```python
from build123d import *

# Parameters (mm, degrees)
SKETCH1_W               = 60
SKETCH1_H               = 40
BOSS_EXTRUDE1_DEPTH     = 27
SKETCH2_W               = 8
SKETCH2_H               = 3
CUT_EXTRUDE1_DEPTH      = 1
CUT_EXTRUDE1_DRAFT      = -35
MIRROR1_COPY_1_SKETCH_W = 8
MIRROR1_COPY_1_SKETCH_H = 3
MIRROR1_COPY_1_DEPTH    = 1
MIRROR1_COPY_1_DRAFT    = -35
MIRROR2_COPY_1_SKETCH_W = 8
MIRROR2_COPY_1_SKETCH_H = 3
MIRROR2_COPY_1_DEPTH    = 1
MIRROR2_COPY_1_DRAFT    = -35
MIRROR2_COPY_2_SKETCH_W = 8
MIRROR2_COPY_2_SKETCH_H = 3
MIRROR2_COPY_2_DEPTH    = 1
MIRROR2_COPY_2_DRAFT    = -35
BOSS_EXTRUDE2_START     = 27
SKETCH1_3_W             = 60
SKETCH1_3_H             = 40
BOSS_EXTRUDE2_DEPTH     = 2
SKETCH3_W               = 21.960696684
SKETCH3_H               = 27.5
CUT_EXTRUDE2_DEPTH      = 2
SKETCH3_3_R             = 2.5
SKETCH3_3_R_2           = 1.4
SKETCH3_3_R_3           = 2.519651658
BOSS_EXTRUDE3_DEPTH     = 5
SKETCH4_W               = 20
SKETCH4_H               = 27
BOSS_EXTRUDE4_DEPTH     = 8
CHAMFER1_SIZE           = 5
CHAMFER1_SIZE_2         = 8.660254038
SKETCH5_W               = 8
SKETCH5_H               = 20
CUT_EXTRUDE3_DEPTH      = 25
SKETCH6_W               = 12
SKETCH6_H               = 40
CUT_EXTRUDE5_DEPTH      = 1.5


with BuildPart() as part:
    # Sketch1 → Boss-Extrude1 (new body)
    with BuildSketch(Plane(origin=(0, 0, 0), x_dir=(1, 0, 0), z_dir=(0, 1, 0))):
        Polygon((-32, 22), (-20, 22), (-20, 21), (-12, 21), (-12, 22), (12, 22), (12, 21), (20, 21), (20, 22), (32, 22), (32, -22), (20, -22), (20, -21), (12, -21), (12, -22), (-12, -22), (-12, -21), (-20, -21), (-20, -22), (-32, -22), align=None)
        Rectangle(SKETCH1_W, SKETCH1_H, mode=Mode.SUBTRACT)
    extrude(amount=BOSS_EXTRUDE1_DEPTH)


with BuildPart() as cut_extrude1_tool:
    # Sketch2 → Cut-Extrude1 (with draft: the straight prism first)
    with BuildSketch(Plane.XY.offset(21)):
        with Locations((-16, 5.5)):
            Rectangle(SKETCH2_W, SKETCH2_H)
    extrude(amount=-CUT_EXTRUDE1_DEPTH)
    # Cut-Extrude1: the draft: its side faces are tilted about the plane it starts from
    cut_extrude1_sides = [cut_extrude1_tool.faces().sort_by_distance(p)[0] for p in [
        (-20, 5.5, 20.5),
        (-16, 4, 20.5),
        (-12, 5.5, 20.5),
        (-16, 7, 20.5),
    ]]
    draft(cut_extrude1_sides, Plane.XY.offset(21), CUT_EXTRUDE1_DRAFT)


with BuildPart() as part_1:
    add(part.part)

    # Cut-Extrude1: cut by cut_extrude1_tool
    add(cut_extrude1_tool.part, mode=Mode.SUBTRACT)


with BuildPart() as mirror1_copy_1_tool:
    # Mirror1 copy 1 sketch → Mirror1 copy 1 (with draft: the straight prism first)
    with BuildSketch(Plane(origin=(0, 0, 21), x_dir=(-1, 0, 0), z_dir=(0, 0, 1))):
        with Locations((-16, -5.5)):
            Rectangle(MIRROR1_COPY_1_SKETCH_W, MIRROR1_COPY_1_SKETCH_H)
    extrude(amount=-MIRROR1_COPY_1_DEPTH)
    # Mirror1 copy 1: the draft: its side faces are tilted about the plane it starts from
    mirror1_copy_1_sides = [mirror1_copy_1_tool.faces().sort_by_distance(p)[0] for p in [
        (20, 5.5, 20.5),
        (16, 4, 20.5),
        (12, 5.5, 20.5),
        (16, 7, 20.5),
    ]]
    draft(mirror1_copy_1_sides, Plane(origin=(0, 0, 21), x_dir=(-1, 0, 0), z_dir=(0, 0, 1)), MIRROR1_COPY_1_DRAFT)


with BuildPart() as part_2:
    add(part_1.part)

    # Mirror1 copy 1: cut by mirror1_copy_1_tool
    add(mirror1_copy_1_tool.part, mode=Mode.SUBTRACT)


with BuildPart() as mirror2_copy_1_tool:
    # Mirror2 copy 1 sketch → Mirror2 copy 1 (with draft: the straight prism first)
    with BuildSketch(Plane(origin=(0, 0, -21), x_dir=(1, 0, 0), z_dir=(0, 0, -1))):
        with Locations((-16, -5.5)):
            Rectangle(MIRROR2_COPY_1_SKETCH_W, MIRROR2_COPY_1_SKETCH_H)
    extrude(amount=-MIRROR2_COPY_1_DEPTH)
    # Mirror2 copy 1: the draft: its side faces are tilted about the plane it starts from
    mirror2_copy_1_sides = [mirror2_copy_1_tool.faces().sort_by_distance(p)[0] for p in [
        (-20, 5.5, -20.5),
        (-16, 4, -20.5),
        (-12, 5.5, -20.5),
        (-16, 7, -20.5),
    ]]
    draft(mirror2_copy_1_sides, Plane(origin=(0, 0, -21), x_dir=(1, 0, 0), z_dir=(0, 0, -1)), MIRROR2_COPY_1_DRAFT)


with BuildPart() as part_3:
    add(part_2.part)

    # Mirror2 copy 1: cut by mirror2_copy_1_tool
    add(mirror2_copy_1_tool.part, mode=Mode.SUBTRACT)


with BuildPart() as mirror2_copy_2_tool:
    # Mirror2 copy 2 sketch → Mirror2 copy 2 (with draft: the straight prism first)
    with BuildSketch(Plane(origin=(0, 0, -21), x_dir=(-1, 0, 0), z_dir=(0, 0, -1))):
        with Locations((-16, 5.5)):
            Rectangle(MIRROR2_COPY_2_SKETCH_W, MIRROR2_COPY_2_SKETCH_H)
    extrude(amount=-MIRROR2_COPY_2_DEPTH)
    # Mirror2 copy 2: the draft: its side faces are tilted about the plane it starts from
    mirror2_copy_2_sides = [mirror2_copy_2_tool.faces().sort_by_distance(p)[0] for p in [
        (20, 5.5, -20.5),
        (16, 4, -20.5),
        (12, 5.5, -20.5),
        (16, 7, -20.5),
    ]]
    draft(mirror2_copy_2_sides, Plane(origin=(0, 0, -21), x_dir=(-1, 0, 0), z_dir=(0, 0, -1)), MIRROR2_COPY_2_DRAFT)


with BuildPart() as part_4:
    add(part_3.part)

    # Mirror2 copy 2: cut by mirror2_copy_2_tool
    add(mirror2_copy_2_tool.part, mode=Mode.SUBTRACT)

    # Sketch1<3> → Boss-Extrude2 (add)
    with BuildSketch(Plane(origin=(0, 0, 0), x_dir=(1, 0, 0), z_dir=(0, 1, 0)).offset(BOSS_EXTRUDE2_START)):
        Rectangle(SKETCH1_3_W, SKETCH1_3_H)
    extrude(amount=-BOSS_EXTRUDE2_DEPTH)

    # Sketch3 → Cut-Extrude2 (cut)
    with BuildSketch(Plane.XZ.offset(-25)):
        with Locations((0.5, 4.25)):
            Rectangle(SKETCH3_W, SKETCH3_H)
    extrude(amount=-CUT_EXTRUDE2_DEPTH, mode=Mode.SUBTRACT)

    # Sketch3<3> → Boss-Extrude3 (add)
    # profile 1 of 4: a face of its own
    with BuildSketch(Plane.XZ.offset(-25)):
        with Locations(Location((-13, 15.25, 0), (0, 0, 90))):
            Circle(SKETCH3_3_R)
        with Locations(Location((-13, 15.25, 0), (0, 0, 270))):
            Circle(SKETCH3_3_R_2, mode=Mode.SUBTRACT)
    # profile 2 of 4: a face of its own
    with BuildSketch(Plane.XZ.offset(-25)):
        with Locations((-13, -6.75)):
            Circle(SKETCH3_3_R_3)
        with Locations(Location((-13, -6.75, 0), (0, 0, 270))):
            Circle(SKETCH3_3_R_2, mode=Mode.SUBTRACT)
    # profile 3 of 4: a face of its own
    with BuildSketch(Plane.XZ.offset(-25)):
        with Locations(Location((14, -6.75, 0), (0, 0, 180))):
            Circle(SKETCH3_3_R_3)
        with Locations(Location((14, -6.75, 0), (0, 0, 270))):
            Circle(SKETCH3_3_R_2, mode=Mode.SUBTRACT)
    # profile 4 of 4: a face of its own
    with BuildSketch(Plane.XZ.offset(-25)):
        with Locations(Location((14, 15.25, 0), (0, 0, 90))):
            Circle(SKETCH3_3_R)
        with Locations(Location((14, 15.25, 0), (0, 0, 270))):
            Circle(SKETCH3_3_R_2, mode=Mode.SUBTRACT)
    extrude(amount=BOSS_EXTRUDE3_DEPTH)

    # Sketch4 → Boss-Extrude4 (add)
    with BuildSketch(Plane(origin=(32, 0, 0), x_dir=(0, 0, -1), z_dir=(1, 0, 0))):
        with Locations((10, 13.5)):
            Rectangle(SKETCH4_W, SKETCH4_H)
    extrude(amount=BOSS_EXTRUDE4_DEPTH)

    # Chamfer1
    # the kernel refuses this chamfer: 8.660254038, 5 mm, written as the material it adds along each edge
    with BuildSketch(Plane(origin=(32, 27, -20), x_dir=(-0.05789386240267251, 0, -0.9983227437537924), z_dir=(0, -1, 0))) as chamfer1_piece_1_section:
        Polygon((CHAMFER1_SIZE * 0.998322743754, CHAMFER1_SIZE * 0.0578938624027), (-CHAMFER1_SIZE_2 * 0.0578938624016, CHAMFER1_SIZE_2 * 0.998322743736), (0, 0), align=None)
    chamfer1_piece_1 = extrude(amount=27, mode=Mode.PRIVATE)
    chamfer1_piece_1 = split(chamfer1_piece_1, bisect_by=Plane(origin=(35.513912711, 13.5, -22), z_dir=(0, 0, 1)), keep=Keep.TOP, mode=Mode.PRIVATE)
    chamfer1_piece_1 = split(chamfer1_piece_1, bisect_by=Plane(origin=(40, 13.5, -20.824917772), z_dir=(-1, 0, 0)), keep=Keep.TOP, mode=Mode.PRIVATE)
    add(chamfer1_piece_1)
    with BuildSketch(Plane(origin=(32, 0, 0), x_dir=(-0.05789386240267113, 0, 0.9983227437537926), z_dir=(0, 1, 0))) as chamfer1_piece_2_section:
        Polygon((CHAMFER1_SIZE * 0.998322743754, CHAMFER1_SIZE * 0.0578938624027), (-CHAMFER1_SIZE_2 * 0.0578938624016, CHAMFER1_SIZE_2 * 0.998322743736), (0, 0), align=None)
    chamfer1_piece_2 = extrude(amount=27, mode=Mode.PRIVATE)
    chamfer1_piece_2 = split(chamfer1_piece_2, bisect_by=Plane(origin=(40, 13.5, 1.631661659), z_dir=(-1, 0, 0)), keep=Keep.TOP, mode=Mode.PRIVATE)
    add(chamfer1_piece_2)

    # Sketch5 → Cut-Extrude3 (cut)
    with BuildSketch(Plane.XZ):
        with Locations((34, -10)):
            Rectangle(SKETCH5_W, SKETCH5_H)
    extrude(amount=-CUT_EXTRUDE3_DEPTH, mode=Mode.SUBTRACT)

    # Sketch6 → Cut-Extrude5 (cut)
    with BuildSketch(Plane.XZ.offset(-25)):
        with Locations((24, 0)):
            Rectangle(SKETCH6_W, SKETCH6_H)
    extrude(amount=-CUT_EXTRUDE5_DEPTH, mode=Mode.SUBTRACT)


solid = part_4.part
```
Geometry check sheet. Reference: the model listing, model coordinates, mm. A direction names the side the tool comes from. Give positions to 0.01 mm unless a question says otherwise; leave off trailing zeros. Order: outer loops, then holes, each group sorted by start corner. A loop starts at its lowest first (then second) coordinate and runs counter-clockwise, first axis right, second up.
1. Release check for a two-part mould opening along X. For faces 4 (the face through (13.89, 22.535, 12.752)), 5 (the face through (40, 13, -10)), 6 (the face through (28, 14, -22)) record: pulls with the +X half, pulls with the -X half, needs draft (parallel to the pull), parting line crosses it, or undercut.
2. Section check B-B, the plane x = 14. Give the number of separate pieces and of enclosed holes in the cut face, and give its area (3 significant figures).
3. Access from +Z, -Z, +X, -X, +Y, -Y to the whole of each face (thin tool, end or side, straight path). Record for faces 1 (the face through (16, 2, -21)), 2 (the face through (38, 12, -10)), 3 (the face through (16, 2, 21)).
4. Thickness scan on L1, parallel to X at y = 19, z = 15.5; L2, parallel to X at y = 23.25, z = -14.5; L3, parallel to Z at x = -6.5, y = 8.75. Record the ranges inside material, lowest first.
5. Section check D-D, the plane z = 8. Enter the section's corners in (x, y), and give its area (3 significant figures).
6. Gauge pin test, flat ends, axial feed: pin 1 Ø10 at (y, z) = (19.5, 3) entering from +X; pin 2 Ø3 at (x, z) = (-12.5, -6.5) entering from -Y; pin 3 Ø2 at (x, y) = (16, 3) entering from +Z; pin 4 Ø6 at (y, z) = (10, 12) entering from +X. Record the tip position at first contact, or that the pin passes through.
Values follow:
1. face 4: undercut
1. face 5: pulls with the +X half
1. face 6: needs draft
2. separate pieces: 3
2. enclosed holes: 0
2. area: 152 mm2
3. face 1: -Z, +Y, -Y
3. face 2: -Y
3. face 3: +Z, +Y, -Y
4. L1: x = -32 to -30, 30 to 32
4. L2: x = -32 to -30, 38 to 40
4. L3: z = -22 to -20, 20 to 22
5. outline: (-32, 0) - (-30, 0) - (-30, 25) - (-10.48, 25) - (-10.48, 27) - (-32, 27) - close; (11.48, 25) - (18, 25) - (18, 26.5) - (30, 26.5) - (30, 0) - (32, 0) - (32, 27) - (11.48, 27) - close
5. area: 166 mm2
6. pin 1: stops at x = 40
6. pin 2: stops at y = 20
6. pin 3: stops at z = 21
6. pin 4: stops at x = 32
